```python
from build123d import *

# Parameters (mm, degrees)
F0_R           = 34.985
F0_R_2         = 26.5
F1_DEPTH       = 32.5
F3_DEPTH       = 23.4
F5_DEPTH       = 18.5
F6_R           = 2.95
F7_R           = 0.8
F8_DEPTH       = 34.9860001
F8_DEPTH_BACK  = 34.9860001
F10_DEPTH      = 9.4
F11_R          = 2.949
F12_R          = 0.8
F13_DEPTH      = 34.9860001
F13_DEPTH_BACK = 34.861403497


# Not quite as in the source:
# - a fillet or chamfer is up to 0.001 mm smaller than in the source, because OpenCascade refuses the exact size


with BuildPart() as f1:
    # F0 (on Top) → F1 (new body)
    with BuildSketch(Plane.XY):
        Circle(F0_R)
        Circle(F0_R_2, mode=Mode.SUBTRACT)
    extrude(amount=F1_DEPTH)

    # F2 (on face) → F3 (cut)
    with BuildSketch(Plane(origin=(0, 0, 0), x_dir=(1, 0, 0), z_dir=(0, 0, -1))):
        with BuildLine():
            ThreePointArc((15.025, 31.5942969537), (0, 34.985), (-15.025, 31.5942969537))
            Line((-15.025, 31.5942969537), (-15.025, 21.828865637))
            ThreePointArc((-15.025, 21.828865637), (0, 26.5), (15.025, 21.828865637))
            Line((15.025, 21.828865637), (15.025, 31.5942969537))
        make_face()
    extrude(amount=-F3_DEPTH, mode=Mode.SUBTRACT)

    # F4 (on face) → F5 (cut)
    with BuildSketch(Plane.XY.offset(32.5)):
        with BuildLine():
            ThreePointArc((34.985, 0), (34.9538369699, 1.4763150336), (34.860403397, 2.95))
            Line((34.860403397, 2.95), (32.5, 2.95))
            Line((32.5, 2.95), (32.5, -2.95))
            Line((32.5, -2.95), (34.860403397, -2.95))
            ThreePointArc((34.860403397, -2.95), (34.9538369699, -1.4763150336), (34.985, 0))
        make_face()
        with BuildLine():
            Line((-32.5, 2.95), (-34.860403397, 2.95))
            ThreePointArc((-34.860403397, 2.95), (-34.985, 0), (-34.860403397, -2.95))
            Line((-34.860403397, -2.95), (-32.5, -2.95))
            Line((-32.5, -2.95), (-32.5, 2.95))
        make_face()
    extrude(amount=-F5_DEPTH, mode=Mode.SUBTRACT)

    # F6
    f6_edges = [f1.edges().sort_by_distance(p)[0] for p in [
        (-33.680202, -2.95, 14),
        (33.680202, 2.95, 14),
    ]]
    fillet(f6_edges, radius=F6_R)

    # F7 (on Right) → F8 (cut, two sides)
    with BuildSketch(Plane.YZ) as f8_sk:
        with Locations((0, 29.5)):
            Circle(F7_R)
    extrude(amount=-F8_DEPTH, mode=Mode.SUBTRACT)
    extrude(f8_sk.sketch, amount=F8_DEPTH_BACK, mode=Mode.SUBTRACT)

    # F9 (on face) → F10 (cut)
    with BuildSketch(Plane.XY.offset(32.5)):
        with BuildLine():
            ThreePointArc((2.95, 34.860403397), (0, 34.985), (-2.95, 34.860403397))
            Line((-2.95, 34.860403397), (-2.95, 32.5))
            Line((-2.95, 32.5), (2.95, 32.5))
            Line((2.95, 32.5), (2.95, 34.860403397))
        make_face()
        with BuildLine():
            Line((-2.95, -32.5), (-2.95, -34.860403397))
            ThreePointArc((-2.95, -34.860403397), (0, -34.985), (2.95, -34.860403397))
            Line((2.95, -34.860403397), (2.95, -32.5))
            Line((2.95, -32.5), (-2.95, -32.5))
        make_face()
    extrude(amount=-F10_DEPTH, mode=Mode.SUBTRACT)

    # F11 (radius 2.95 in the source; OpenCascade refuses exactly that, so slightly less here)
    f11_edges = [f1.edges().sort_by_distance(p)[0] for p in [
        (-2.95, 33.680202, 23.1),
        (2.95, 33.680202, 23.1),
    ]]
    fillet(f11_edges, radius=F11_R)

    # F12 (on Front) → F13 (cut, two sides)
    with BuildSketch(Plane.XZ) as f13_sk:
        with Locations((0, 26)):
            Circle(F12_R)
    extrude(amount=-F13_DEPTH, mode=Mode.SUBTRACT)
    extrude(f13_sk.sketch, amount=F13_DEPTH_BACK, mode=Mode.SUBTRACT)


solid = f1.part
```
Geometry check sheet. Reference: the model listing, model coordinates, mm. A direction names the side the tool comes from. Round coordinates to 2 decimals unless told otherwise and drop trailing zeros. Order: outer loops, then holes, each group sorted by start corner. A loop starts at its lowest first (then second) coordinate and runs counter-clockwise, first axis right, second up. Notation, with made-up numbers: (13, 1) - (17, 1) arc R9 ccw to (17, 8) - close; hole circle Ø1 at (-19, 55.5). An arc over 180 degrees is marked (long way). Use a Markdown table: item, result. Add a question column.
(1) Material ranges on line 1 along Z through (x, y) = (0, -31); line 2 along X through (y, z) = (0, 28); line 3 along Z through (x, y) = (0, 29.5), recorded low to high. Write a range as [from, to].
(2) Sectioned sample at C-C, the plane z = 8. Enter the section's corners in (x, y) (3 decimals).
(3) Depth check by flat-ended pin: pin 1 (5 mm diameter, centred on y = -11.5, z = 22.5, fed in from -X); pin 2 (1.5 mm diameter, centred on y = 1, z = 16, fed in from -X); pin 3 (10 mm diameter, centred on y = 21, z = 20.5, fed in from +X). Enter the tip coordinate at first touch or a pass-through.
(4) Tool access check on faces 1 (the flat face through (0, -32.5, 28)), 2 (the cylindrical face through (-2.11, 33.73, 23.99)), 3 (the flat face through (-15.025, -27, 12)), 4 (the cylindrical face through (33.73, 2.06, 14.84)), 5 (the flat face through (-32.5, 0, 23)). Record the directions out of +Z, -Z, +X, -X, +Y, -Y that give a thin tool (end or side, any length) a straight path to the whole face; none if there is none.
(5) Sectioned sample at B-B, the plane y = 16. Enter the section's corners in (x, z).
(6) Sectioned sample at D-D, the plane x = 31.5. Enter the section's corners in (y, z), and give its area (3 significant figures).
(7) Sectioned sample at A-A, the plane x = -4.5. Enter the section's corners in (y, z).
(8) Release check for a two-part mould opening along Y. For faces 6 (the flat face through (0, 32.5, 28)), 7 (the cylindrical face through (-20.8, 28.13, 16.02)), 8 (the flat face through (15, -23, 32.5)), 9 (the cylindrical face through (-3.45, 26.274, 16.022)) record: pulls with the +Y half, pulls with the -Y half, needs draft (parallel to the pull), parting line crosses it, or undercut.
Answers below:
| question | item | result |
|---|---|---|
| 1 | line 1 | [23.4, 25.2], [26.8, 32.5] |
| 1 | line 2 | [-32.5, -26.5], [26.5, 32.5] |
| 1 | line 3 | [0, 25.2], [26.8, 32.5] |
| 2 | outline | (-15.025, -31.594) - (-15.025, -21.829) arc R26.5 cw (long way) to (15.025, -21.829) - (15.025, -31.594) arc R34.985 ccw (long way) to start |
| 3 | pin 1 | x = -33.81 |
| 3 | pin 2 | x = -32.5 |
| 3 | pin 3 | x = 31.11 |
| 4 | face 1 | +Z, -Z, -Y |
| 4 | face 2 | +Z, +Y |
| 4 | face 3 | -Z, -Y |
| 4 | face 4 | +Z, +X |
| 4 | face 5 | +Z, -X |
| 5 | outline | (-31.11, 0) - (-21.12, 0) - (-21.12, 32.5) - (-31.11, 32.5) - close; (21.12, 0) - (31.11, 0) - (31.11, 32.5) - (21.12, 32.5) - close |
| 6 | outline | (-15.22, 0) - (15.22, 0) - (15.22, 32.5) - (-15.22, 32.5) - close; hole circle Ø1.6 at (0, 29.5) |
| 6 | area | 987 mm² |
| 7 | outline | (-34.69, 23.4) - (-26.12, 23.4) - (-26.12, 32.5) - (-34.69, 32.5) - close; (26.12, 0) - (34.69, 0) - (34.69, 32.5) - (26.12, 32.5) - close |
| 8 | face 6 | pulls with the +Y half |
| 8 | face 7 | parting line crosses it |
| 8 | face 8 | needs draft |
| 8 | face 9 | undercut |
